from build123d import *

# Parameters (mm, degrees)
RESSALTO_EXTRUS_O1_DEPTH   = 19.8
ESBO_O3_R                  = 1.6
CORTE_EXTRUS_O1_DEPTH      = 3
CORTE_EXTRUS_O2_REACH      = 38.62
CORTE_EXTRUS_O2_END_RADIUS = 45
ESBO_O4_R                  = 3.15


with BuildPart() as part:
    # Esboço1 → Ressalto-extrusão1 (new body)
    with BuildSketch(Plane.XY):
        with BuildLine():
            Line((-25, 37.416573868), (-25, 32.996573868))
            Line((-25, 32.996573868), (-15, 32.996573868))
            Line((-15, 32.996573868), (-15, 17.996573868))
            Line((-15, 17.996573868), (15, 17.996573868))
            Line((15, 17.996573868), (15, 32.996573868))
            Line((15, 32.996573868), (25, 32.996573868))
            Line((25, 32.996573868), (25, 37.416573868))
            ThreePointArc((25, 37.416573868), (0, 45), (-25, 37.416573868))
        make_face()
    extrude(amount=RESSALTO_EXTRUS_O1_DEPTH)

    # Esboço3 → Corte-extrusão1 (cut)
    with BuildSketch(Plane.XZ.offset(-32.996573868)):
        with Locations(Location((21, 9.8, 0), (0, 0, 270))):
            Circle(ESBO_O3_R)
        with Locations(Location((-21, 9.8, 0), (0, 0, 270))):
            Circle(ESBO_O3_R)
    extrude(amount=-CORTE_EXTRUS_O1_DEPTH, mode=Mode.SUBTRACT)

    # Corte-extrusão2: up to this cylinder (the profile starts inside it)
    corte_extrus_o2_end = Plane(origin=(0, 0, 9.8), z_dir=(0, 0, -1)) * Cylinder(CORTE_EXTRUS_O2_END_RADIUS, 168.24, mode=Mode.PRIVATE)
    # Esboço4 → Corte-extrusão2 (cut, up to the surface)
    with BuildSketch(Plane.XZ.offset(-35.996573868), mode=Mode.PRIVATE) as corte_extrus_o2_sk1:
        with Locations(Location((21, 9.8, 0), (0, 0, 270))):
            Circle(ESBO_O4_R)
    corte_extrus_o2_tool1 = extrude(corte_extrus_o2_sk1.sketch, amount=-CORTE_EXTRUS_O2_REACH, mode=Mode.PRIVATE) & corte_extrus_o2_end
    add(corte_extrus_o2_tool1.solids().sort_by_distance((21, 35.996574, 9.8))[0], mode=Mode.SUBTRACT)
    # Esboço4 → Corte-extrusão2 (cut, up to the surface)
    with BuildSketch(Plane.XZ.offset(-35.996573868), mode=Mode.PRIVATE) as corte_extrus_o2_sk2:
        with Locations(Location((-21, 9.8, 0), (0, 0, 270))):
            Circle(ESBO_O4_R)
    corte_extrus_o2_tool2 = extrude(corte_extrus_o2_sk2.sketch, amount=-CORTE_EXTRUS_O2_REACH, mode=Mode.PRIVATE) & corte_extrus_o2_end
    add(corte_extrus_o2_tool2.solids().sort_by_distance((-21, 35.996574, 9.8))[0], mode=Mode.SUBTRACT)


solid = part.part
Design review of the part built by this model. Coordinates are the model's own, in mm. A direction names the side the tool comes from. Round coordinates to 2 decimals unless told otherwise and drop trailing zeros. Write each loop counter-clockwise with the first axis right and the second up, starting at its lowest first coordinate (ties: lowest second). Pieces come first, ordered by that corner, then holes. Notation, with made-up numbers: (62, -10.5) -> (95, -10.5) arc R21 cw to (95, 7.5) -> close; hole circle Ø11 at (46.25, -11.75). An arc over 180 degrees is marked (long way). One line per item, written item: value. Start each with the question number.
Q1. Insertion check: P1, Ø4, axis at y = 28.5, z = 9, coming from the -X side; P2, Ø8, axis at x = -20.5, z = 8.5, coming from the -Y side; P3, Ø3, axis at x = -21, z = 9, coming from the +Y side. Each pin has a flat end and moves straight along its axis. Give the tip position at first contact, or say it passes through.
Q2. Add section A-A (z = 8.75). Give the boundary of the cut face in (x, y).
Q3. To check wall thickness, follow probe 1 along X at (y, z) = (34, 9.8); probe 2 along Z at (x, y) = (-21, 38.9); probe 3 along X at (y, z) = (25.25, 12.75). State the ranges of each line that lie inside material, in increasing order.
Q4. Tool access review of faces 4 (the face through (15, 25, 10)), 5 (the face through (-17.877, 38.031, 10.21)), 6 (the face through (-19, 32.997, 10)): name each direction out of +Z, -Z, +X, -X, +Y, -Y from which nothing blocks a thin tool from reaching the whole face with its end or side.
Q5. The part is to be moulded in two halves that separate along X. For faces 1 (the face through (0, 45, 10)), 2 (the face through (-22, 35.997, 8)), 3 (the face through (0, 17.997, 10)), say which applies: pulls with the +X half, pulls with the -X half, needs draft (parallel to the pull), parting line crosses it, or undercut.
Q6. Add section C-C (x = -21). Give the boundary of the cut face in (y, z), then the cut area to 3 significant figures.
Q7. Add section B-B (z = 15.25). Give the boundary of the cut face in (x, y).
Q8. Add section D-D (y = 38.5). Give the boundary of the cut face in (x, z), then the cut area to 3 significant figures.
Response:
1. P1: stops at x = -15
1. P2: stops at y = 33
1. P3: stops at y = 36
2. outline: (-25, 33) -> (-22.21, 33) -> (-22.21, 36) -> (-23.97, 36) -> (-23.97, 38.08) arc R45 ccw to (-25, 37.42) -> close; (-19.79, 33) -> (-15, 33) -> (-15, 18) -> (15, 18) -> (15, 33) -> (19.79, 33) -> (19.79, 36) -> (18.03, 36) -> (18.03, 41.23) arc R45 ccw to (-18.03, 41.23) -> (-18.03, 36) -> (-19.79, 36) -> close; (22.21, 33) -> (25, 33) -> (25, 37.42) arc R45 ccw to (23.97, 38.08) -> (23.97, 36) -> (22.21, 36) -> close
3. probe 1: x = -25 to -22.6, -19.4 to 19.4, 22.6 to 25
3. probe 2: z = 0 to 6.65, 12.95 to 19.8
3. probe 3: x = -15 to 15
4. face 4: +Z, -Z, +X, -Y
4. face 5: +Y
4. face 6: +Z, -Z, -X, -Y
5. face 1: parting line crosses it
5. face 2: undercut
5. face 3: needs draft
6. outline: (33, 0) -> (39.8, 0) -> (39.8, 6.65) -> (36, 6.65) -> (36, 8.2) -> (33, 8.2) -> close; (33, 11.4) -> (36, 11.4) -> (36, 12.95) -> (39.8, 12.95) -> (39.8, 19.8) -> (33, 19.8) -> close
6. area: 101 mm^2
7. outline: (-25, 33) -> (-15, 33) -> (-15, 18) -> (15, 18) -> (15, 33) -> (25, 33) -> (25, 37.42) arc R45 ccw to (-25, 37.42) -> close
8. outline: (-23.3, 0) -> (23.3, 0) -> (23.3, 7.64) arc R3.15 cw (long way) to (23.3, 11.96) -> (23.3, 19.8) -> (-23.3, 19.8) -> (-23.3, 11.96) arc R3.15 cw (long way) to (-23.3, 7.64) -> close
8. area: 865 mm^2
